Source: CAD feature listing. Evaluate the final solid. Frame: model axes, mm. A direction names the side the tool comes from. Coordinates: 2 decimals unless noted, no trailing zeros. Order: outer loops, then holes, each group sorted by start corner. A loop starts at its lowest first (then second) coordinate and runs counter-clockwise, first axis right, second up. Notation, with made-up numbers: (46.5, 50) -> (98.5, 50) arc R15 ccw to (98.5, 58) -> close; hole circle Ø8 at (52.25, 6). An arc over 180 degrees is marked (long way). Write item = value, one per line. Start each with the question number.
Item 1: Section query B-B (y = -4). Output: boundary loops of the cut face in (x, z).
Item 2: Ray query, line 1 along Z through (x, y) = (-108.5, -32.5); line 2 along Z through (x, y) = (-106.5, -17); line 3 along Y through (x, z) = (-105.5, -18.4). Return the intervals inside material, ascending. Write a range as [from, to].
Item 3: Set-up query: faces 4 (the flat face through (-106, 2, -15)), 5 (the flat face through (-106, -25.108, -15)). Return all of +Z, -Z, +X, -X, +Y, -Y with unobstructed straight access to the full face (end or side cutting, diameter ignored); none if empty.
Item 4: Mould query, pull axis Z, two halves, no side actions, for faces 1 (the flat face through (-106, -22, -9.681)), 2 (the cylindrical face through (-105.76, -28.417, -8.852)), 3 (the cylindrical face through (-105.94, -37.43, -8.6)). Classes: released by +Z, released by -Z, zero draft, split by the parting line, or undercut.
Item 5: Section query A-A (x = -105.5). Output: boundary loops of the cut face in (y, z).
Item 6: Section query C-C (z = -16). Output: boundary loops of the cut face in (x, y).
Item 7: Section query D-D (y = -30.4). Output: boundary loops of the cut face in (x, z).
```python
from build123d import *

# Parameters (mm, degrees)
CYLINDER009_R     = 2
CYLINDER009_DEPTH = 50
PAD001_DEPTH      = 30
CYLINDER008_R     = 1.8
CYLINDER008_DEPTH = 50
BOX006_W          = 10
BOX006_H          = 40
BOX006_DEPTH      = 14
FILLET_R          = 2


with BuildPart() as cylinder009:
    # Cylinder009 → Cylinder009 (new body)
    with BuildSketch(Plane(origin=(-105.5, -30.4, -37), x_dir=(1, 0, 0), z_dir=(0, 0, 1))):
        Circle(CYLINDER009_R)
    extrude(amount=CYLINDER009_DEPTH)


with BuildPart() as body001:
    # Sketch001 → Pad001 (new body)
    with BuildSketch(Plane.YZ):
        Polygon((-34.905251, -9.681131), (-8.889799, -9.681131), (-8.889799, -13.181131), (-25.107943, -13.181131), (-25.107943, -16.681131), (-34.905251, -16.681131), align=None)
    extrude(amount=PAD001_DEPTH)


with BuildPart() as body001_1:
    # Body001 placement: moved
    add(body001.part.moved(Location((-110, 0, 0))))


with BuildPart() as fusion001005:
    # Cylinder008 → Cylinder008 (new body)
    with BuildSketch(Plane(origin=(-143, -4, -16), x_dir=(0, 0, -1), z_dir=(1, 0, 0))):
        Circle(CYLINDER008_R)
    extrude(amount=CYLINDER008_DEPTH)

    # Fusion001005: union Cylinder009, Body001
    add(cylinder009.part)
    add(body001_1.part)


with BuildPart() as fillet_body:
    # Box006 → Box006 (new body)
    with BuildSketch(Plane(origin=(-112, -38, -22), x_dir=(1, 0, 0), z_dir=(0, 0, 1))):
        with Locations((5, 20)):
            Rectangle(BOX006_W, BOX006_H)
    extrude(amount=BOX006_DEPTH)

    # Cut009: cut Fusion001005
    add(fusion001005.part, mode=Mode.SUBTRACT)

    # Fillet
    fillet_edges = [fillet_body.edges().sort_by_distance(p)[0] for p in [
        (-112, -38, -15),
        (-112, -18, -8),
        (-112, -18, -22),
        (-112, 2, -15),
        (-107, -38, -22),
        (-107, -38, -8),
        (-107, 2, -8),
        (-107, 2, -22),
    ]]
    fillet(fillet_edges, radius=FILLET_R)


solid = fillet_body.part
```
Computed:
q1.outline = (-112, -20) arc R2 ccw to (-110, -22) -> (-102, -22) -> (-102, -17.8) -> (-112, -17.8) -> close; (-112, -14.2) -> (-102, -14.2) -> (-102, -8) -> (-110, -8) arc R2 ccw to (-112, -10) -> close
q2.line_1 = [-22, -16.68], [-9.68, -8]
q2.line_2 = [-22, -13.18], [-9.68, -8]
q2.line_3 = [-38, -32.4], [-28.4, 2]
q3.face_4 = +Z, -Z, +X, -X, +Y
q3.face_5 = +X
q4.face_1 = undercut
q4.face_2 = zero draft
q4.face_3 = released by +Z
q5.outline = (-38, -20) arc R2 ccw to (-36, -22) -> (-32.4, -22) -> (-32.4, -16.68) -> (-34.91, -16.68) -> (-34.91, -9.68) -> (-32.4, -9.68) -> (-32.4, -8) -> (-36, -8) arc R2 ccw to (-38, -10) -> close; (-28.4, -22) -> (0, -22) arc R2 ccw to (2, -20) -> (2, -10) arc R2 ccw to (0, -8) -> (-28.4, -8) -> (-28.4, -9.68) -> (-8.89, -9.68) -> (-8.89, -13.18) -> (-25.11, -13.18) -> (-25.11, -16.68) -> (-28.4, -16.68) -> close; hole circle Ø3.6 at (-4, -16)
q6.outline = (-112, -36) arc R2 ccw to (-110, -38) -> (-102, -38) -> (-102, -34.91) -> (-110, -34.91) -> (-110, -25.11) -> (-102, -25.11) -> (-102, -5.8) -> (-112, -5.8) -> close; (-112, -2.2) -> (-102, -2.2) -> (-102, 2) -> (-110, 2) arc R2 ccw to (-112, 0) -> close
q7.outline = (-112, -20) arc R2 ccw to (-110, -22) -> (-107.5, -22) -> (-107.5, -16.68) -> (-110, -16.68) -> (-110, -9.68) -> (-107.5, -9.68) -> (-107.5, -8) -> (-110, -8) arc R2 ccw to (-112, -10) -> close; (-103.5, -22) -> (-102, -22) -> (-102, -16.68) -> (-103.5, -16.68) -> close; (-103.5, -9.68) -> (-102, -9.68) -> (-102, -8) -> (-103.5, -8) -> close
